Here's how the part is built. I have some questions about the finished solid (model axes, mm). Face numbers are marked on the shaded views. A direction names the side the tool comes from. Round coordinates to 2 decimals unless told otherwise and drop trailing zeros. Order: outer loops, then holes, each group sorted by start corner. A loop starts at its lowest first (then second) coordinate and runs counter-clockwise, first axis right, second up. Notation, with made-up numbers: (29, 38.25) -> (44, 38.25) arc R15 ccw to (44, 52.25) -> close; hole circle Ø2 at (-38.75, -39). An arc over 180 degrees is marked (long way). One line per item, written item: value.
```python
from build123d import *

# Parameters (mm, degrees)
F0_W     = 50
F0_H     = 65
F1_DEPTH = 6
F2_W     = 28
F2_H     = 40
F3_DEPTH = 25
F4_R     = 1.55
F5_DEPTH = 10
F6_R     = 1.55
F7_DEPTH = 10


with BuildPart() as f1:
    # F0 (on Top) → F1 (new body)
    with BuildSketch(Plane.XY):
        Rectangle(F0_W, F0_H)
    extrude(amount=F1_DEPTH)

    # F2 (on face) → F3 (cut)
    with BuildSketch(Plane.XY.offset(6)):
        Rectangle(F2_W, F2_H)
    extrude(amount=-F3_DEPTH, mode=Mode.SUBTRACT)

    # F4 (on face) → F5 (cut)
    with BuildSketch(Plane.YZ.offset(25)):
        with BuildLine():
            ThreePointArc((-30.05, 3), (-28.5, 1.45), (-26.95, 3))
            ThreePointArc((-26.95, 3), (-28.5, 4.55), (-30.05, 3))
        make_face()
        with Locations((28.5, 3)):
            Circle(F4_R)
    extrude(amount=-F5_DEPTH, mode=Mode.SUBTRACT)

    # F6 (on face) → F7 (cut)
    with BuildSketch(Plane(origin=(-25, 0, 0), x_dir=(0, -1, 0), z_dir=(-1, 0, 0))):
        with BuildLine():
            ThreePointArc((-30.05, 3), (-28.5, 1.45), (-26.95, 3))
            ThreePointArc((-26.95, 3), (-28.5, 4.55), (-30.05, 3))
        make_face()
        with Locations((28.5, 3)):
            Circle(F6_R)
    extrude(amount=-F7_DEPTH, mode=Mode.SUBTRACT)


solid = f1.part
```
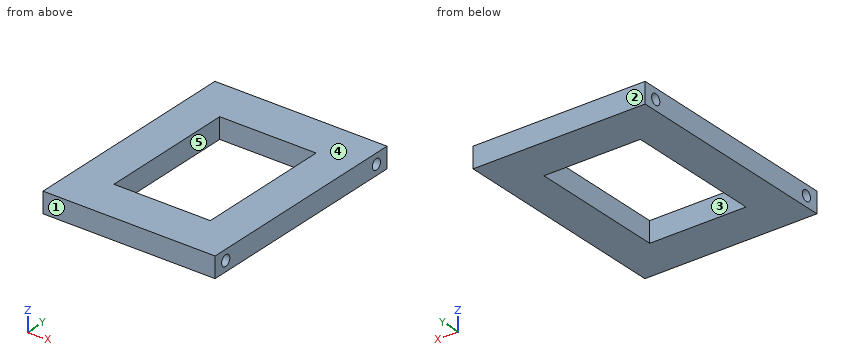
Q1. For P1, Ø3.5, axis at y = -29, z = 3.5, coming from the -X side; P2, Ø1.9, axis at y = 28.5, z = 3, coming from the -X side; P3, Ø2.5, axis at y = -28.5, z = 3, coming from the +X side, each with a flat end and sliding along its axis, tell me the tip position at first contact or that it passes through.
Answers:
P1: x = -25
P2: x = -15
P3: x = 15
Q2. If we mould it in two halves opening along Y, with no side actions, what happens to the marked faces 1, 2 and 3? For each: pulls with the +Y half, pulls with the -Y half, needs draft (parallel to the pull), parting line crosses it, or undercut.
Answers:
face 1: pulls with the -Y half
face 2: pulls with the +Y half
face 3: undercut
Q3. I want a section at C-C on y = 28.5. Write out the boundary of the cut face in (x, z), then the cut area to 3 significant figures.
Answers:
outline: (-25, 0) -> (25, 0) -> (25, 1.45) -> (15, 1.45) -> (15, 4.55) -> (25, 4.55) -> (25, 6) -> (-25, 6) -> (-25, 4.55) -> (-15, 4.55) -> (-15, 1.45) -> (-25, 1.45) -> close
area: 238 mm2
Q4. I need wall thicknesses on line 1 along X through (y, z) = (14, 2.95); line 2 along Y through (x, z) = (-2, 4.4); line 3 along Z through (x, y) = (-22, 28.5). Which ranges of each line are inside material? Lowest first, please.
Answers:
line 1: -25 to -14, 14 to 25
line 2: -32.5 to -20, 20 to 32.5
line 3: 0 to 1.45, 4.55 to 6
Q5. I want a section at B-B on z = 3. Write out the boundary of the cut face in (x, y), then the cut area to 3 significant figures.
Answers:
outline: (-25, -32.5) -> (25, -32.5) -> (25, -30.05) -> (15, -30.05) -> (15, -26.95) -> (25, -26.95) -> (25, 26.95) -> (15, 26.95) -> (15, 30.05) -> (25, 30.05) -> (25, 32.5) -> (-25, 32.5) -> (-25, 30.05) -> (-15, 30.05) -> (-15, 26.95) -> (-25, 26.95) -> (-25, -26.95) -> (-15, -26.95) -> (-15, -30.05) -> (-25, -30.05) -> close; hole (-14, -20) -> (14, -20) -> (14, 20) -> (-14, 20) -> close
area: 2,010 mm2
Q6. I want a section at D-D on y = 14. Write out the boundary of the cut face in (x, z).
Answers:
outline: (-25, 0) -> (-14, 0) -> (-14, 6) -> (-25, 6) -> close; (14, 0) -> (25, 0) -> (25, 6) -> (14, 6) -> close
Q7. Which directions (+Z, -Z, +X, -X, +Y, -Y) give clear straight access to the entire face, cutting with the end or side of a thin tool? Please do the marked faces 4 and 5.
Answers:
face 4: +Z, +X, -X, +Y, -Y
face 5: +Z, -Z
Q8. I want a section at A-A on x = 3. Write out the boundary of the cut face in (y, z).
Answers:
outline: (-32.5, 0) -> (-20, 0) -> (-20, 6) -> (-32.5, 6) -> close; (20, 0) -> (32.5, 0) -> (32.5, 6) -> (20, 6) -> close
